Check sheet for the modelled part. Datum: model origin and axes. Units: mm. Give positions to 0.01 mm unless a question says otherwise; leave off trailing zeros. Order: outer loops, then holes, each group sorted by start corner. A loop starts at its lowest first (then second) coordinate and runs counter-clockwise, first axis right, second up. Notation, with made-up numbers: (-29.5, 83.5) -> (29.5, 83.5) arc R31 ccw to (29.5, 112.5) -> close; hole circle Ø4 at (61.25, -22). An arc over 180 degrees is marked (long way). Write each question's results on one line, items separated by ' | '.
from build123d import *

# Parameters (mm, degrees)
SKETCH1_R             = 1.89865
BOSS_EXTRUDE1_DEPTH   = 12.7
FILLET1_R             = 1.5875
F_6_CLEARANCE_HOLE1_D = 3.7973


with BuildPart() as part:
    # Sketch1 → Boss-Extrude1 (new body)
    with BuildSketch(Plane.XY):
        with BuildLine():
            Line((-17.318712187, -0.508773921), (-11.1125, -6.35))
            Line((-11.1125, -6.35), (11.1125, -6.35))
            Line((11.1125, -6.35), (17.318712187, -0.508773921))
            ThreePointArc((17.318712187, -0.508773921), (18.287874783, 3.844327942), (14.59865, 6.35))
            Line((14.59865, 6.35), (12.7, 6.35))
            Line((12.7, 6.35), (-12.7, 6.35))
            Line((-12.7, 6.35), (-14.59865, 6.35))
            ThreePointArc((-14.59865, 6.35), (-18.287874783, 3.844327942), (-17.318712187, -0.508773921))
        make_face()
        with Locations((-14.59865, 2.38125)):
            Circle(SKETCH1_R, mode=Mode.SUBTRACT)
    extrude(amount=BOSS_EXTRUDE1_DEPTH)

    # Fillet1
    fillet1_edges = [part.edges().sort_by_distance(p)[0] for p in [
        (11.1125, -6.35, 6.35),
        (-11.1125, -6.35, 6.35),
    ]]
    fillet(fillet1_edges, radius=FILLET1_R)

    # #6 Clearance Hole1 (through all)
    with Locations(Plane.XY.offset(12.7)):
        with Locations((-14.59865, 2.38125), (14.59865, 2.38125)):
            Hole(F_6_CLEARANCE_HOLE1_D / 2)


solid = part.part
1. Gauge pin test, flat ends, axial feed: pin 1 Ø6 at (x, y) = (14.6, 2.38) entering from -Z; pin 2 Ø3 at (y, z) = (-2, 10.5) entering from -X; pin 3 Ø4 at (y, z) = (-5, 10.5) entering from -X; pin 4 Ø3.5 at (x, y) = (-14.6, 2.38) entering from -Z. Record the tip position at first contact, or that the pin passes through.
Verdict:
pin 1: stops at z = 0 | pin 2: stops at x = -17.33 | pin 3: stops at x = -14.67 | pin 4: passes through
2. Section check D-D on y = 5.25. Record the cut outline in (x, z).
Verdict:
outline: (-17.34, 0) -> (17.34, 0) -> (17.34, 12.7) -> (-17.34, 12.7) -> close
3. Mould release check, pull along X, two halves, no side actions. Record for faces 1 (the flat face through (-14.485, -3.176, 6.261)), 2 (the flat face through (14.405, -3.252, 6.261)), 3 (the flat face through (0, 6.35, 6)), 4 (the cylindrical face through (-12.845, 1.654, 6.261)): +X half, -X half, draft (parallel to the pull), parting line (faces both ways), or undercut.
Verdict:
face 1: -X half | face 2: +X half | face 3: draft | face 4: undercut
4. Section check A-A on y = 3. Record the cut outline in (x, z), then the cut area to 3 significant figures.
Verdict:
outline: (-18.52, 0) -> (-16.39, 0) -> (-16.39, 12.7) -> (-18.52, 12.7) -> close; (-12.8, 0) -> (12.8, 0) -> (12.8, 12.7) -> (-12.8, 12.7) -> close; (16.39, 0) -> (18.52, 0) -> (18.52, 12.7) -> (16.39, 12.7) -> close | area: 379 mm^2
5. Section check C-C on y = -4. Record the cut outline in (x, z), then the cut area to 3 significant figures.
Verdict:
outline: (-13.61, 0) -> (13.61, 0) -> (13.61, 12.7) -> (-13.61, 12.7) -> close | area: 346 mm^2
6. Material ranges on probe 1 along X at (y, z) = (2.5, 1.75); probe 2 along X at (y, z) = (3.25, 9.5); probe 3 along Y at (x, z) = (14.5, 3.25), recorded low to high. Write a range as from..to.
Verdict:
probe 1: x = -18.57..-16.49, -12.7..12.7, 16.49..18.57 | probe 2: x = -18.47..-16.29, -12.91..12.91, 16.29..18.47 | probe 3: y = -3.16..0.49, 4.28..6.35
7. Section check B-B on z = 7.25. Give the number of separate pieces and of enclosed holes in the cut face, then the cut area to 3 significant figures.
Verdict:
separate pieces: 1 | enclosed holes: 2 | area: 389 mm^2
